```python
from build123d import *

# Parameters (mm, degrees)
BOSS_EXTRUDE1_DEPTH = 3.175


with BuildPart() as part:
    # Sketch1 → Boss-Extrude1 (new body)
    with BuildSketch(Plane.XY):
        Polygon((0, 0), (80, 0), (80, 55), (76.825, 55), (76.825, 135), (80, 135), (80, 205), (76.825, 205), (76.825, 235), (40, 235), (40, 231.825), (0, 231.825), (-40, 231.825), (-40, 235), (-76.825, 235), (-76.825, 205), (-80, 205), (-80, 135), (-76.825, 135), (-76.825, 55), (-80, 55), (-80, 0), align=None)
    extrude(amount=-BOSS_EXTRUDE1_DEPTH)


solid = part.part
```
Design review of the part built by this model. Coordinates are the model's own, in mm. Coordinates: 2 decimals unless noted, no trailing zeros. Order: outer loops, then holes, each group sorted by start corner. A loop starts at its lowest first (then second) coordinate and runs counter-clockwise, first axis right, second up.
1) Take a section at A-A, the plane z = -1.7. Give the boundary of the cut face in (x, y) (3 decimals).
2) Take a section at B-B, the plane y = 109. Give the boundary of the cut face in (x, z) (3 decimals).
3) Wall thickness on line 1 along Y through (x, z) = (21, -2.05) (3 decimals); line 2 along X through (y, z) = (209.5, -2.65) (3 decimals): over which ranges is each line inside the solid? List them lowest first.
4) Clearance check with flat-ended pins moving along their axes: pin 1 (1 mm diameter, centred on x = 46.5, y = 198.5, fed in from +Z); pin 2 (1.6 mm diameter, centred on x = 78.5, z = -1, fed in from +Y); pin 3 (1 mm diameter, centred on x = 4, z = -1.5, fed in from +Y) (3 decimals); pin 4 (1.5 mm diameter, centred on y = 98, z = -2, fed in from +X) (3 decimals). State where each tip first meets the part, or that it passes through.
Returned:
1. outline: (-80, 0) - (80, 0) - (80, 55) - (76.825, 55) - (76.825, 135) - (80, 135) - (80, 205) - (76.825, 205) - (76.825, 235) - (40, 235) - (40, 231.825) - (-40, 231.825) - (-40, 235) - (-76.825, 235) - (-76.825, 205) - (-80, 205) - (-80, 135) - (-76.825, 135) - (-76.825, 55) - (-80, 55) - close
2. outline: (-76.825, -3.175) - (76.825, -3.175) - (76.825, 0) - (-76.825, 0) - close
3. line 1: y = 0 to 231.825
3. line 2: x = -76.825 to 76.825
4. pin 1: stops at z = 0
4. pin 2: stops at y = 205
4. pin 3: stops at y = 231.825
4. pin 4: stops at x = 76.825
